Source: CAD feature listing. Evaluate the final solid. Frame: model axes, mm. A direction names the side the tool comes from. Round coordinates to 2 decimals unless told otherwise and drop trailing zeros. Order: outer loops, then holes, each group sorted by start corner. A loop starts at its lowest first (then second) coordinate and runs counter-clockwise, first axis right, second up. Notation, with made-up numbers: (25, 88.25) -> (82, 88.25) arc R31 cw to (82, 115.25) -> close; hole circle Ø1 at (-20.75, 80.5). An arc over 180 degrees is marked (long way). One line per item, written item: value. Start each with the question number.
1) Pin query (flat end, axial travel): P1, Ø4, axis at y = 16.5, z = 41, coming from the -X side; P2, Ø1.2, axis at x = -20, y = -48, coming from the +Z side; P3, Ø14, axis at y = -6.37, z = 81.32, coming from the +X side; P4, Ø6, axis at x = -25, y = -31, coming from the +Z side. Return the tip coordinate at first contact, or that it passes through.
2) Ray query, L1, parallel to X at y = -32, z = 71; L2, parallel to Y at x = -39, z = 11; L3, parallel to Z at x = -24, y = -34.5. Return the intervals inside material, ascending.
3) Section C-C (y = 41). Return the cut outline in (x, z).
4) Section A-A (x = -55). Return the cut outline in (y, z), and give its area (4 significant figures).
5) Reachability of faces 4 (the face through (-68.16, -33.82, 85.74)), 5 (the face through (28.071, 0, 40)) from +Z, -Z, +X, -X, +Y, -Y: full face, straight path, thin tool, end or side. Return the list, or none.
6) Section B-B (y = -24). Return the cut outline in (x, z), and give its area (3 significant figures).
7) Mould query, pull axis Z, two halves, no side actions, for faces 1 (the face through (-20, 2, 2.5)), 2 (the face through (29.339, -4.094, 39.973)), 3 (the face through (-20, -48.853, 25)). Classes: pulls with the +Z half, pulls with the -Z half, needs draft (parallel to the pull), parting line crosses it, or undercut.
```python
from build123d import *

# Parameters (mm, degrees)
F0_W     = 100
F0_H     = 100
F1_DEPTH = 100
F2_T     = -2.5
F3_W     = 94.5649716185
F3_H     = 2.5
F4_DEPTH = 50
F5_R     = 50
F6_R     = 12.0743721724
F6_R_2   = 11.213441631
F6_R_3   = 12.3428155876
F6_R_4   = 11.6683976529
F6_R_5   = 10.6581459458
F6_R_6   = 12.1539399679
F7_DEPTH = 100.001


with BuildPart() as f1:
    # F0 (on Top) → F1 (new body)
    with BuildSketch(Plane.XY):
        with Locations((-19.4285236971, 1.1470969766)):
            Rectangle(F0_W, F0_H)
    extrude(amount=F1_DEPTH)

    # F2
    f2_openings = [f1.faces().sort_by_distance(p)[0] for p in [
        (-19.428524, 1.147097, 100),
    ]]
    offset(amount=F2_T, openings=f2_openings)

    # F3 (on face) → F4 (cut)
    with BuildSketch(Plane.XY.offset(100)):
        with Locations((-19.6460378879, -47.6029030234)):
            Rectangle(F3_W, F3_H)
    extrude(amount=-F4_DEPTH, mode=Mode.SUBTRACT)

    # F5
    f5_edges = [f1.edges().sort_by_distance(p)[0] for p in [
        (-68.178524, -48.852903, 100),
        (29.103962, -48.852903, 100),
    ]]
    fillet(f5_edges, radius=F5_R)

    # F6 (on face) → F7 (cut, through all)
    with BuildSketch(Plane.YZ.offset(30.5714763029)):
        with Locations((-28.1003583223, 53.0040338635)):
            Circle(F6_R)
        with Locations((-2.6344081853, 28.8552865386)):
            Circle(F6_R_2)
        with Locations((0, 53.8821704686)):
            Circle(F6_R_3)
        with Locations((-6.3664885238, 81.323929131)):
            Circle(F6_R_4)
        with Locations((26.3440869749, 73.6402347684)):
            Circle(F6_R_5)
        with Locations((26.3440869749, 46.1984761059)):
            Circle(F6_R_6)
    extrude(amount=-F7_DEPTH, mode=Mode.SUBTRACT)


solid = f1.part
```
Findings:
1. P1: x = -69.43
1. P2: z = 50
1. P3: through
1. P4: z = 2.5
2. L1: -69.43 to -66.93, 28.07 to 30.57
2. L2: -48.85 to -46.35, 48.65 to 51.15
2. L3: 0 to 2.5
3. outline: (-69.43, 0) -> (30.57, 0) -> (30.57, 100) -> (28.07, 100) -> (28.07, 2.5) -> (-66.93, 2.5) -> (-66.93, 100) -> (-69.43, 100) -> close
4. outline: (-48.85, 0) -> (51.15, 0) -> (51.15, 100) -> (48.65, 100) -> (48.65, 2.5) -> (-46.35, 2.5) -> (-46.35, 50) -> (-48.85, 50) -> close
4. area: 612.5 mm2
5. face 4: +Z, +X, -X, -Y
5. face 5: +Z
6. outline: (-69.43, 0) -> (30.57, 0) -> (30.57, 41.65) -> (28.07, 41.65) -> (28.07, 2.5) -> (-66.93, 2.5) -> (-66.93, 41.65) -> (-69.43, 41.65) -> close; (-69.43, 64.36) -> (-66.93, 64.36) -> (-66.93, 93.22) -> (-69.43, 93.22) -> close; (28.07, 64.36) -> (30.57, 64.36) -> (30.57, 93.22) -> (28.07, 93.22) -> close
6. area: 590 mm2
7. face 1: pulls with the +Z half
7. face 2: undercut
7. face 3: needs draft
